from build123d import *

# Parameters (mm, degrees)
F0_R     = 700
F1_DEPTH = 2
F2_R     = 700
F2_R_2   = 699
F3_DEPTH = 50
F4_R     = 6
F5_DEPTH = 300


with BuildPart() as f1:
    # F0 (on Top) → F1 (new body)
    with BuildSketch(Plane.XY):
        Circle(F0_R)
    extrude(amount=F1_DEPTH)

    # F2 (on face) → F3 (join)
    with BuildSketch(Plane(origin=(0, 0, 0), x_dir=(1, 0, 0), z_dir=(0, 0, -1))):
        Circle(F2_R)
        Circle(F2_R_2, mode=Mode.SUBTRACT)
    extrude(amount=F3_DEPTH)

    # F4 (on face) → F5 (join)
    with BuildSketch(Plane(origin=(0, 0, 0), x_dir=(1, 0, 0), z_dir=(0, 0, -1))):
        with Locations((-150, 0)):
            Circle(F4_R)
        with Locations((0, 150)):
            Circle(F4_R)
        with Locations((150, 0)):
            Circle(F4_R)
        with Locations((0, -150)):
            Circle(F4_R)
    extrude(amount=F5_DEPTH)


solid = f1.part
CAD build for the part. Positions are in the model's coordinates, mm. Give positions to 0.01 mm unless a question says otherwise; leave off trailing zeros. Write each loop counter-clockwise with the first axis right and the second up, starting at its lowest first coordinate (ties: lowest second). Pieces come first, ordered by that corner, then holes. Notation, with made-up numbers: M 67.5,74.5 L 93.5,74.5 A25 ccw 93.5,93.5 Z; hole C -13,12.25 d6. An arc over 180 degrees is marked long. Put each result on its own line as item: value. Start each with the question number.
(1) Probe L1, parallel to X at y = 0, z = -9.5; L2, parallel to Z at x = -249, y = -279. List the from-to ranges inside material, lowest first.
(2) Band-saw the part on A-A, the plane z = -31. Write the cut outline in (x, y), and give its area (3 significant figures).
(3) Band-saw the part on B-B, the plane x = -228.5. Write the cut outline in (y, z), and give its area (3 significant figures).
(4) Band-saw the part on C-C, the plane y = -351.5. Write the cut outline in (x, z), and give its area (3 significant figures).
(5) Mould opens along Y. For faces 1 (the face through (-515.93, -473.09, -23.64)), 2 (the face through (-10, 10, 2)), 3 (the face through (666.72, -209.96, -24.65)) say: +Y half, -Y half, draft (parallel to the pull), parting line (faces both ways), or undercut.
(6) Flat gauge pins, fed straight in: pin 1 Ø12 at (y, z) = (-545.5, -50) entering from +X; pin 2 Ø6 at (y, z) = (126, -44.5) entering from -X. Where does each tip first touch, or does it go through?
(7) Band-saw the part on D-D, the plane z = -272. Write the cut outline in (x, y).
Response values:
1. L1: x = -700 to -699, -156 to -144, 144 to 156, 699 to 700
1. L2: z = 0 to 2
2. outline: C 0,0 d1400; C -150,0 d12; C 0,-150 d12; C 0,150 d12; C 150,0 d12; hole C 0,0 d1398
2. area: 4,850 mm2
3. outline: M -661.66,-50 L -660.6,-50 L -660.6,0 L 660.6,0 L 660.6,-50 L 661.66,-50 L 661.66,2 L -661.66,2 Z
3. area: 2,750 mm2
4. outline: M -605.35,-50 L -604.19,-50 L -604.19,0 L 604.19,0 L 604.19,-50 L 605.35,-50 L 605.35,2 L -605.35,2 Z
4. area: 2,540 mm2
5. face 1: parting line
5. face 2: draft
5. face 3: undercut
6. pin 1: stops at x = 446.03
6. pin 2: stops at x = -689.11
7. outline: C -150,0 d12; C 0,-150 d12; C 0,150 d12; C 150,0 d12
